Can you work these out from the model? Positions are in its coordinate system, mm. Round coordinates to 2 decimals unless told otherwise and drop trailing zeros. Loops run counter-clockwise (first coordinate to the right, second up) from the corner with the lowest first, then second, coordinate; pieces in that order, holes last.
(1) Will this pin go through, and if not, where does the flat tip stop? pin 1 Ø3.5 at (x, z) = (-25, -30) entering from -Y.
(2) I want a section at A-A on z = 30. Give the number of separate pieces and of enclosed holes in the cut face, plus the area to 3 significant figures.
(3) If I drill on line 1 along Z through (x, y) = (76.5, 2), over which ranges is the centre line in solid material (lowest first)?
(4) I want a section at B-B on x = 75. Write out the boundary of the cut face in (y, z), plus the area to 3 significant figures.
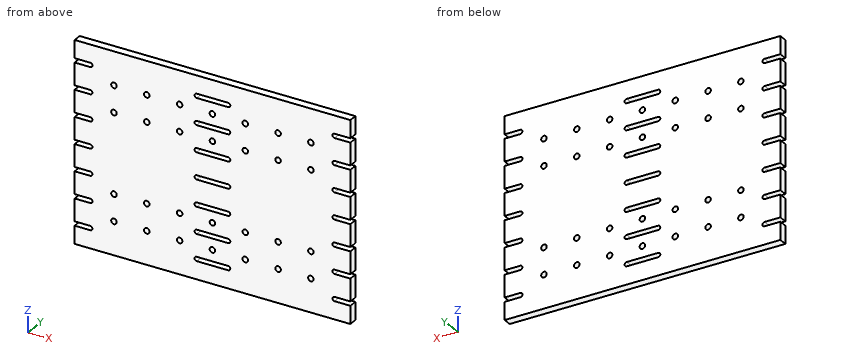
from build123d import *

# Parameters (mm, degrees)
SKETCH1_W                  = 210
SKETCH1_H                  = 150
BOSS_EXTRUDE1_DEPTH        = 6.35
CUT_EXTRUDE1_DEPTH         = 130.191031035
LPATTERN1_COUNT            = 4
LPATTERN1_PITCH            = 20
LPATTERN1_COL_COUNT        = 4
LPATTERN1_COL_PITCH        = 20
LPATTERN2_COUNT            = 2
LPATTERN2_PITCH            = 105
LPATTERN2_COPY_1_DEPTH     = 130.191031035
LPATTERN2_COPY_2_DEPTH     = 130.191031035
LPATTERN2_COPY_3_DEPTH     = 130.191031035
LPATTERN2_COPY_4_DEPTH     = 130.191031035
LPATTERN2_COPY_5_DEPTH     = 130.191031035
LPATTERN2_COPY_6_DEPTH     = 130.191031035
LPATTERN2_COL_COUNT        = 2
LPATTERN2_COL_PITCH        = 105
LPATTERN2_COL_COPY_1_DEPTH = 130.191031035
LPATTERN2_COL_COPY_2_DEPTH = 130.191031035
LPATTERN2_COL_COPY_3_DEPTH = 130.191031035
LPATTERN2_COL_COPY_4_DEPTH = 130.191031035
LPATTERN2_COL_COPY_5_DEPTH = 130.191031035
LPATTERN2_COL_COPY_6_DEPTH = 130.191031035
SKETCH4_R                  = 2.1
CUT_EXTRUDE2_DEPTH         = 130.191031035
LPATTERN3_COUNT            = 4
LPATTERN3_PITCH            = 25
LPATTERN3_COL_COUNT        = 4
LPATTERN3_COL_PITCH        = 25


with BuildPart() as part:
    # Sketch1 → Boss-Extrude1 (new body)
    with BuildSketch(Plane(origin=(0, 0, 0), x_dir=(1, 0, 0), z_dir=(0, 1, 0))):
        Rectangle(SKETCH1_W, SKETCH1_H)
    extrude(amount=BOSS_EXTRUDE1_DEPTH)

    # Sketch3 → Cut-Extrude1 (cut, symmetric)
    with BuildSketch(Plane(origin=(0, 6.35, 0), x_dir=(1, 0, 0), z_dir=(0, 1, 0))):
        with BuildLine():
            Line((12, -1.6), (-12, -1.6))
            ThreePointArc((-12, -1.6), (-13.6, 0), (-12, 1.6))
            Line((-12, 1.6), (12, 1.6))
            ThreePointArc((12, 1.6), (13.6, 0), (12, -1.6))
        make_face()
    cut_extrude1 = extrude(amount=CUT_EXTRUDE1_DEPTH, both=True, mode=Mode.SUBTRACT)

    # LPattern1: Cut-Extrude1 ×4
    with Locations(*[(0, 0, i * LPATTERN1_PITCH) for i in range(1, LPATTERN1_COUNT)]):
        add(cut_extrude1, mode=Mode.SUBTRACT)

    # LPattern1 col: Cut-Extrude1 ×4
    with Locations(*[(0, 0, -i * LPATTERN1_COL_PITCH) for i in range(1, LPATTERN1_COL_COUNT)]):
        add(cut_extrude1, mode=Mode.SUBTRACT)

    # LPattern2: Cut-Extrude1 ×2
    with Locations(*[(i * LPATTERN2_PITCH, 0, 0) for i in range(1, LPATTERN2_COUNT)]):
        add(cut_extrude1, mode=Mode.SUBTRACT)

    # LPattern2 copy 1 sketch → LPattern2 copy 1 (cut, symmetric)
    with BuildSketch(Plane(origin=(105, 6.35, 20), x_dir=(1, 0, 0), z_dir=(0, 1, 0))):
        with BuildLine():
            Line((12, -1.6), (-12, -1.6))
            ThreePointArc((-12, -1.6), (-13.6, 0), (-12, 1.6))
            Line((-12, 1.6), (12, 1.6))
            ThreePointArc((12, 1.6), (13.6, 0), (12, -1.6))
        make_face()
    extrude(amount=LPATTERN2_COPY_1_DEPTH, both=True, mode=Mode.SUBTRACT)

    # LPattern2 copy 2 sketch → LPattern2 copy 2 (cut, symmetric)
    with BuildSketch(Plane(origin=(105, 6.35, 40), x_dir=(1, 0, 0), z_dir=(0, 1, 0))):
        with BuildLine():
            Line((12, -1.6), (-12, -1.6))
            ThreePointArc((-12, -1.6), (-13.6, 0), (-12, 1.6))
            Line((-12, 1.6), (12, 1.6))
            ThreePointArc((12, 1.6), (13.6, 0), (12, -1.6))
        make_face()
    extrude(amount=LPATTERN2_COPY_2_DEPTH, both=True, mode=Mode.SUBTRACT)

    # LPattern2 copy 3 sketch → LPattern2 copy 3 (cut, symmetric)
    with BuildSketch(Plane(origin=(105, 6.35, 60), x_dir=(1, 0, 0), z_dir=(0, 1, 0))):
        with BuildLine():
            Line((12, -1.6), (-12, -1.6))
            ThreePointArc((-12, -1.6), (-13.6, 0), (-12, 1.6))
            Line((-12, 1.6), (12, 1.6))
            ThreePointArc((12, 1.6), (13.6, 0), (12, -1.6))
        make_face()
    extrude(amount=LPATTERN2_COPY_3_DEPTH, both=True, mode=Mode.SUBTRACT)

    # LPattern2 copy 4 sketch → LPattern2 copy 4 (cut, symmetric)
    with BuildSketch(Plane(origin=(105, 6.35, -20), x_dir=(1, 0, 0), z_dir=(0, 1, 0))):
        with BuildLine():
            Line((12, -1.6), (-12, -1.6))
            ThreePointArc((-12, -1.6), (-13.6, 0), (-12, 1.6))
            Line((-12, 1.6), (12, 1.6))
            ThreePointArc((12, 1.6), (13.6, 0), (12, -1.6))
        make_face()
    extrude(amount=LPATTERN2_COPY_4_DEPTH, both=True, mode=Mode.SUBTRACT)

    # LPattern2 copy 5 sketch → LPattern2 copy 5 (cut, symmetric)
    with BuildSketch(Plane(origin=(105, 6.35, -40), x_dir=(1, 0, 0), z_dir=(0, 1, 0))):
        with BuildLine():
            Line((12, -1.6), (-12, -1.6))
            ThreePointArc((-12, -1.6), (-13.6, 0), (-12, 1.6))
            Line((-12, 1.6), (12, 1.6))
            ThreePointArc((12, 1.6), (13.6, 0), (12, -1.6))
        make_face()
    extrude(amount=LPATTERN2_COPY_5_DEPTH, both=True, mode=Mode.SUBTRACT)

    # LPattern2 copy 6 sketch → LPattern2 copy 6 (cut, symmetric)
    with BuildSketch(Plane(origin=(105, 6.35, -60), x_dir=(1, 0, 0), z_dir=(0, 1, 0))):
        with BuildLine():
            Line((12, -1.6), (-12, -1.6))
            ThreePointArc((-12, -1.6), (-13.6, 0), (-12, 1.6))
            Line((-12, 1.6), (12, 1.6))
            ThreePointArc((12, 1.6), (13.6, 0), (12, -1.6))
        make_face()
    extrude(amount=LPATTERN2_COPY_6_DEPTH, both=True, mode=Mode.SUBTRACT)

    # LPattern2 col: Cut-Extrude1 ×2
    with Locations(*[(-i * LPATTERN2_COL_PITCH, 0, 0) for i in range(1, LPATTERN2_COL_COUNT)]):
        add(cut_extrude1, mode=Mode.SUBTRACT)

    # LPattern2 col copy 1 sketch → LPattern2 col copy 1 (cut, symmetric)
    with BuildSketch(Plane(origin=(-105, 6.35, 20), x_dir=(1, 0, 0), z_dir=(0, 1, 0))):
        with BuildLine():
            Line((12, -1.6), (-12, -1.6))
            ThreePointArc((-12, -1.6), (-13.6, 0), (-12, 1.6))
            Line((-12, 1.6), (12, 1.6))
            ThreePointArc((12, 1.6), (13.6, 0), (12, -1.6))
        make_face()
    extrude(amount=LPATTERN2_COL_COPY_1_DEPTH, both=True, mode=Mode.SUBTRACT)

    # LPattern2 col copy 2 sketch → LPattern2 col copy 2 (cut, symmetric)
    with BuildSketch(Plane(origin=(-105, 6.35, 40), x_dir=(1, 0, 0), z_dir=(0, 1, 0))):
        with BuildLine():
            Line((12, -1.6), (-12, -1.6))
            ThreePointArc((-12, -1.6), (-13.6, 0), (-12, 1.6))
            Line((-12, 1.6), (12, 1.6))
            ThreePointArc((12, 1.6), (13.6, 0), (12, -1.6))
        make_face()
    extrude(amount=LPATTERN2_COL_COPY_2_DEPTH, both=True, mode=Mode.SUBTRACT)

    # LPattern2 col copy 3 sketch → LPattern2 col copy 3 (cut, symmetric)
    with BuildSketch(Plane(origin=(-105, 6.35, 60), x_dir=(1, 0, 0), z_dir=(0, 1, 0))):
        with BuildLine():
            Line((12, -1.6), (-12, -1.6))
            ThreePointArc((-12, -1.6), (-13.6, 0), (-12, 1.6))
            Line((-12, 1.6), (12, 1.6))
            ThreePointArc((12, 1.6), (13.6, 0), (12, -1.6))
        make_face()
    extrude(amount=LPATTERN2_COL_COPY_3_DEPTH, both=True, mode=Mode.SUBTRACT)

    # LPattern2 col copy 4 sketch → LPattern2 col copy 4 (cut, symmetric)
    with BuildSketch(Plane(origin=(-105, 6.35, -20), x_dir=(1, 0, 0), z_dir=(0, 1, 0))):
        with BuildLine():
            Line((12, -1.6), (-12, -1.6))
            ThreePointArc((-12, -1.6), (-13.6, 0), (-12, 1.6))
            Line((-12, 1.6), (12, 1.6))
            ThreePointArc((12, 1.6), (13.6, 0), (12, -1.6))
        make_face()
    extrude(amount=LPATTERN2_COL_COPY_4_DEPTH, both=True, mode=Mode.SUBTRACT)

    # LPattern2 col copy 5 sketch → LPattern2 col copy 5 (cut, symmetric)
    with BuildSketch(Plane(origin=(-105, 6.35, -40), x_dir=(1, 0, 0), z_dir=(0, 1, 0))):
        with BuildLine():
            Line((12, -1.6), (-12, -1.6))
            ThreePointArc((-12, -1.6), (-13.6, 0), (-12, 1.6))
            Line((-12, 1.6), (12, 1.6))
            ThreePointArc((12, 1.6), (13.6, 0), (12, -1.6))
        make_face()
    extrude(amount=LPATTERN2_COL_COPY_5_DEPTH, both=True, mode=Mode.SUBTRACT)

    # LPattern2 col copy 6 sketch → LPattern2 col copy 6 (cut, symmetric)
    with BuildSketch(Plane(origin=(-105, 6.35, -60), x_dir=(1, 0, 0), z_dir=(0, 1, 0))):
        with BuildLine():
            Line((12, -1.6), (-12, -1.6))
            ThreePointArc((-12, -1.6), (-13.6, 0), (-12, 1.6))
            Line((-12, 1.6), (12, 1.6))
            ThreePointArc((12, 1.6), (13.6, 0), (12, -1.6))
        make_face()
    extrude(amount=LPATTERN2_COL_COPY_6_DEPTH, both=True, mode=Mode.SUBTRACT)

    # Sketch4 → Cut-Extrude2 (cut, symmetric)
    with BuildSketch(Plane(origin=(0, 6.35, 0), x_dir=(1, 0, 0), z_dir=(0, 1, 0))):
        with Locations(Location((0, 30, 0), (0, 0, 270))):
            Circle(SKETCH4_R)
        with Locations(Location((0, -30, 0), (0, 0, 270))):
            Circle(SKETCH4_R)
        with Locations(Location((0, 50, 0), (0, 0, 270))):
            Circle(SKETCH4_R)
        with Locations(Location((0, -50, 0), (0, 0, 270))):
            Circle(SKETCH4_R)
    cut_extrude2 = extrude(amount=CUT_EXTRUDE2_DEPTH, both=True, mode=Mode.SUBTRACT)

    # LPattern3: Cut-Extrude2 ×4
    with Locations(*[(i * LPATTERN3_PITCH, 0, 0) for i in range(1, LPATTERN3_COUNT)]):
        add(cut_extrude2, mode=Mode.SUBTRACT)

    # LPattern3 col: Cut-Extrude2 ×4
    with Locations(*[(-i * LPATTERN3_COL_PITCH, 0, 0) for i in range(1, LPATTERN3_COL_COUNT)]):
        add(cut_extrude2, mode=Mode.SUBTRACT)


solid = part.part
Filled sheet:
1. pin 1: passes through
2. separate pieces: 8
2. enclosed holes: 0
2. area: 1,150 mm2
3. line 1: z = -75 to -51.47, -48.53 to -31.47, -28.53 to 28.53, 31.47 to 48.53, 51.47 to 75
4. outline: (0, -75) - (6.35, -75) - (6.35, -52.1) - (0, -52.1) - close; (0, -47.9) - (6.35, -47.9) - (6.35, -32.1) - (0, -32.1) - close; (0, -27.9) - (6.35, -27.9) - (6.35, 27.9) - (0, 27.9) - close; (0, 32.1) - (6.35, 32.1) - (6.35, 47.9) - (0, 47.9) - close; (0, 52.1) - (6.35, 52.1) - (6.35, 75) - (0, 75) - close
4. area: 846 mm2
